Geometry check sheet. Reference: the model listing, model coordinates, mm. A direction names the side the tool comes from. Give positions to 0.01 mm unless a question says otherwise; leave off trailing zeros. Loops run counter-clockwise (first coordinate to the right, second up) from the corner with the lowest first, then second, coordinate; pieces in that order, holes last. Notation, with made-up numbers: (8, 74) -> (16, 74) arc R26 cw to (16, 113) -> close; hole circle Ø8 at (57, 47). An arc over 180 degrees is marked (long way). One line per item, written item: value. Start each with the question number.
(1) Scan lines: line 1 along Y through (x, z) = (78, 20); line 2 along Z through (x, y) = (58, 40); line 3 along Z through (x, y) = (66, 34.5). Record each from-to range of solid material in increasing order. Write a range as from..to.
(2) Sectioned sample at D-D, the plane y = 27.5. Record the cut outline in (x, z).
(3) Gauge pin test, flat ends, axial feed: pin 1 Ø10 at (y, z) = (74, 56.5) entering from +X; pin 2 Ø24 at (x, y) = (110, 9.5) entering from +Z; pin 3 Ø12 at (x, z) = (62.5, 67.5) entering from +Y. Record the tip position at first contact, or that the pin passes through.
(4) Sectioned sample at B-B, the plane x = 53. Record the cut outline in (y, z).
(5) Sectioned sample at C-C, the plane z = 61.5. Record the cut outline in (x, y), then the cut area to 3 significant figures.
(6) Tool access check on faces 1 (the face through (60, 10, 40)), 2 (the face through (60, 40, 70)), 3 (the face through (60, 70, 40)), 4 (the face through (35, 41, 80)). Record the directions out of +Z, -Z, +X, -X, +Y, -Y that give a thin tool (end or side, any length) a straight path to the whole face; none if there is none.
(7) Sectioned sample at A-A, the plane y = 40. Record the cut outline in (x, z).
(8) Draft check along Y on faces 5 (the face through (56, 60, 55)), 6 (the face through (47.507, 44.614, 11.128)), 7 (the face through (80, 39, 40)). Enter one of: pulls with the +Y half, pulls with the -Y half, needs draft (parallel to the pull), parting line crosses it, or undercut.
from build123d import *

# Parameters (mm, degrees)
F0_W     = 20
F0_H     = 80
F1_DEPTH = 80
F2_DEPTH = 40
F3_DEPTH = 60
F5_DEPTH = 80
F0_W_2   = 40
F0_H_2   = 20
F6_DEPTH = 20
F7_R     = 10
F8_DEPTH = 120


with BuildPart() as f1:
    # F0 (on Top) → F1 (new body)
    with BuildSketch(Plane.XY):
        with Locations((10, 40)):
            Rectangle(F0_W, F0_H)
        Polygon((20, 80), (20, 0), (40, 0), (40, 20), (60, 20), (60, 60), (40, 60), (40, 80), align=None)
    extrude(amount=F1_DEPTH)

    # F0 (on Top) → F2 (join)
    with BuildSketch(Plane.XY):
        Polygon((80, 80), (40, 80), (40, 60), (60, 60), (80, 60), align=None)
        Polygon((40, 20), (40, 0), (80, 0), (80, 20), (60, 20), align=None)
    extrude(amount=F2_DEPTH)

    # F0 (on Top) → F3 (join)
    with BuildSketch(Plane.XY):
        Polygon((60, 20), (80, 20), (80, 30), (80, 50), (80, 60), (60, 60), align=None)
    extrude(amount=F3_DEPTH)

    # F4 (on face) → F5 (cut)
    with BuildSketch(Plane.XZ):
        Polygon((20, 80), (0, 80), (0, 60), align=None)
    extrude(amount=-F5_DEPTH, mode=Mode.SUBTRACT)

    # F0 (on Top) → F6 (join)
    with BuildSketch(Plane.XY):
        Polygon((120, 80), (80, 80), (80, 60), (80, 50), (120, 50), align=None)
        Polygon((80, 20), (80, 0), (120, 0), (120, 30), (80, 30), align=None)
        with Locations((100, 40)):
            Rectangle(F0_W_2, F0_H_2)
    extrude(amount=F6_DEPTH)

    # F7 (on face) → F8 (cut)
    with BuildSketch(Plane.YZ.offset(120)):
        with Locations((40, 20)):
            Circle(F7_R)
    extrude(amount=-F8_DEPTH, mode=Mode.SUBTRACT)


solid = f1.part
Calculated:
1. line 1: y = 0..30, 50..80
1. line 2: z = 0..10, 30..80
1. line 3: z = 0..11.65, 28.35..60
2. outline: (0, 0) -> (120, 0) -> (120, 20) -> (80, 20) -> (80, 60) -> (60, 60) -> (60, 80) -> (20, 80) -> (0, 60) -> close
3. pin 1: stops at x = 40
3. pin 2: stops at z = 20
3. pin 3: stops at y = 60
4. outline: (0, 0) -> (80, 0) -> (80, 40) -> (60, 40) -> (60, 80) -> (20, 80) -> (20, 40) -> (0, 40) -> close; hole circle Ø20 at (40, 20)
5. outline: (1.5, 0) -> (40, 0) -> (40, 20) -> (60, 20) -> (60, 60) -> (40, 60) -> (40, 80) -> (1.5, 80) -> close
5. area: 3,880 mm2
6. face 1: +Z, +X, -Y
6. face 2: +Z, +X, +Y, -Y
6. face 3: +Z, +X, +Y
6. face 4: +Z, +X, -X, +Y, -Y
7. outline: (0, 0) -> (120, 0) -> (120, 10) -> (0, 10) -> close; (0, 30) -> (80, 30) -> (80, 60) -> (60, 60) -> (60, 80) -> (20, 80) -> (0, 60) -> close
8. face 5: pulls with the +Y half
8. face 6: undercut
8. face 7: needs draft
